from build123d import *
from OCP.BRepFilletAPI import BRepFilletAPI_MakeChamfer
from build123d.topology import SkipClean

# Parameters (mm, degrees)
SALIENTE_EXTRUIR1_DEPTH      = 9
CROQUIS3_R                   = 1.344119186
SALIENTE_EXTRUIR2_DEPTH      = 1
CROQUIS4_R                   = 12.5
CROQUIS4_R_2                 = 1.444119186
SALIENTE_EXTRUIR3_DEPTH      = 3
CROQUIS5_R                   = 1.444119186
SALIENTE_EXTRUIR4_DEPTH      = 2
SALIENTE_EXTRUIR5_START      = -3
CROQUIS6_R                   = 1.625
SALIENTE_EXTRUIR5_DEPTH      = 3
CROQUIS7_R                   = 3.125
CROQUIS7_R_2                 = 1.625
SALIENTE_EXTRUIR6_DEPTH      = 1.75
CROQUIS8_R                   = 3.125
CROQUIS8_R_2                 = 1.625
SALIENTE_EXTRUIR7_DEPTH      = 10
SALIENTE_EXTRUIR8_DEPTH      = 13
SALIENTE_EXTRUIR8_DEPTH_BACK = 7
CROQUIS9_R                   = 2.5
REDONDEO1_R                  = 2.5
CROQUIS11_R                  = 2.5
CROQUIS11_R_2                = 1
SALIENTE_EXTRUIR9_DEPTH      = 10
CHAFL_N1_SIZE                = 2
CHAFL_N1_SIZE2               = 1
CROQUIS10_R                  = 1
CORTAR_EXTRUIR1_DEPTH        = 15


with BuildPart() as part:
    # Croquis2 → Saliente-Extruir1 (new body)
    with BuildSketch(Plane.XY):
        with BuildLine():
            Line((-12.5, 12.5), (12.5, 12.5))
            Line((12.5, 12.5), (12.5, 9.5))
            Line((12.5, 9.5), (9.952027427, 7.563540844))
            ThreePointArc((9.952027427, 7.563540844), (12.5, 0), (9.952027427, -7.563540844))
            Line((9.952027427, -7.563540844), (12.5, -9.5))
            Line((12.5, -9.5), (12.5, -12.5))
            Line((12.5, -12.5), (-12.5, -12.5))
            Line((-12.5, -12.5), (-12.5, -9.5))
            Line((-12.5, -9.5), (-9.952027427, -7.563540844))
            ThreePointArc((-9.952027427, -7.563540844), (-12.5, 0), (-9.952027427, 7.563540844))
            Line((-9.952027427, 7.563540844), (-12.5, 9.5))
            Line((-12.5, 9.5), (-12.5, 12.5))
        make_face()
    extrude(amount=SALIENTE_EXTRUIR1_DEPTH)

    # Croquis3 → Saliente-Extruir2 (add)
    with BuildSketch(Plane(origin=(0, 0, 0), x_dir=(-1, 0, 0), z_dir=(0, 0, -1))):
        Circle(CROQUIS3_R)
    extrude(amount=SALIENTE_EXTRUIR2_DEPTH)



with BuildPart() as body_2:
    # Croquis4 → Saliente-Extruir3 (new body)
    with BuildSketch(Plane(origin=(0, 0, 0), x_dir=(-1, 0, 0), z_dir=(0, 0, -1))):
        Circle(CROQUIS4_R)
        Circle(CROQUIS4_R_2, mode=Mode.SUBTRACT)
    extrude(amount=SALIENTE_EXTRUIR3_DEPTH)

    # Croquis5 → Saliente-Extruir4 (add)
    with BuildSketch(Plane(origin=(0, 0, -3), x_dir=(-1, 0, 0), z_dir=(0, 0, -1))):
        Circle(CROQUIS5_R)
    extrude(amount=-SALIENTE_EXTRUIR4_DEPTH)

    # Croquis6 → Saliente-Extruir5 (add)
    # profile 1 of 2: a face of its own
    with BuildSketch(Plane(origin=(0, 0, -3), x_dir=(-1, 0, 0), z_dir=(0, 0, -1)).offset(SALIENTE_EXTRUIR5_START)):
        with BuildLine():
            Line((-12.478662951, 0.73004859), (-16.792901594, -0.118663584))
            ThreePointArc((-16.792901594, -0.118663584), (-19.255933186, -3.788094791), (-15.586501979, -6.251126382))
            Line((-15.586501979, -6.251126382), (-11.272263337, -5.402414208))
            ThreePointArc((-11.272263337, -5.402414208), (-12.264925596, -2.41279923), (-12.478662951, 0.73004859))
        make_face()
        with Locations((-16.189701787, -3.184894983)):
            Circle(CROQUIS6_R, mode=Mode.SUBTRACT)
    # profile 2 of 2: a face of its own
    with BuildSketch(Plane(origin=(0, 0, -3), x_dir=(-1, 0, 0), z_dir=(0, 0, -1)).offset(SALIENTE_EXTRUIR5_START)):
        with BuildLine():
            Line((15.586501979, 6.251126382), (11.272263337, 5.402414208))
            ThreePointArc((11.272263337, 5.402414208), (12.264925596, 2.41279923), (12.478662951, -0.73004859))
            Line((12.478662951, -0.73004859), (16.792901594, 0.118663584))
            ThreePointArc((16.792901594, 0.118663584), (19.255933186, 3.788094791), (15.586501979, 6.251126382))
        make_face()
        with Locations((16.189701787, 3.184894983)):
            Circle(CROQUIS6_R, mode=Mode.SUBTRACT)
    extrude(amount=SALIENTE_EXTRUIR5_DEPTH)

    # Croquis7 → Saliente-Extruir6 (add)
    # profile 1 of 2: a face of its own
    with BuildSketch(Plane(origin=(0, 0, -3), x_dir=(-1, 0, 0), z_dir=(0, 0, -1))):
        with Locations((-16.189701787, -3.184894983)):
            Circle(CROQUIS7_R)
        with Locations((-16.189701787, -3.184894983)):
            Circle(CROQUIS7_R_2, mode=Mode.SUBTRACT)
    # profile 2 of 2: a face of its own
    with BuildSketch(Plane(origin=(0, 0, -3), x_dir=(-1, 0, 0), z_dir=(0, 0, -1))):
        with Locations((16.189701787, 3.184894983)):
            Circle(CROQUIS7_R)
        with Locations((16.189701787, 3.184894983)):
            Circle(CROQUIS7_R_2, mode=Mode.SUBTRACT)
    extrude(amount=SALIENTE_EXTRUIR6_DEPTH)

    # Croquis8 → Saliente-Extruir7 (add)
    # profile 1 of 2: a face of its own
    with SkipClean():  # the faces are left unmerged after this step: merging them gives an invalid solid
        with BuildSketch(Plane.XY):
            with Locations(Location((-16.189701787, 3.184894983, 0), (0, 0, 180))):
                Circle(CROQUIS8_R)
            with Locations(Location((-16.189701787, 3.184894983, 0), (0, 0, 180))):
                Circle(CROQUIS8_R_2, mode=Mode.SUBTRACT)
        # profile 2 of 2: a face of its own
        with BuildSketch(Plane.XY):
            with Locations(Location((16.189701787, -3.184894983, 0), (0, 0, 180))):
                Circle(CROQUIS8_R)
            with Locations(Location((16.189701787, -3.184894983, 0), (0, 0, 180))):
                Circle(CROQUIS8_R_2, mode=Mode.SUBTRACT)
        extrude(amount=SALIENTE_EXTRUIR7_DEPTH)


with BuildPart() as part_1:
    add(part.part)

    add(body_2.part)  # Saliente-Extruir8 merges body 2
    # Croquis9 → Saliente-Extruir8 (add, two sides: drawn at the far end of the back side and taken through both)
    with BuildSketch(Plane(origin=(0, 12.5, 0), x_dir=(1, 0, 0), z_dir=(0, 1, 0)).offset(-SALIENTE_EXTRUIR8_DEPTH_BACK)):
        with Locations(Location((0, -9, 0), (0, 0, 270))):
            Circle(CROQUIS9_R)
    extrude(amount=SALIENTE_EXTRUIR8_DEPTH + SALIENTE_EXTRUIR8_DEPTH_BACK)

    # Redondeo1
    redondeo1_edges = [part_1.edges().sort_by_distance(p)[0] for p in [
        (1.767766953, 5.5, 10.767766953),
    ]]
    fillet(redondeo1_edges, radius=REDONDEO1_R - 0.0001)  # a hair under: the kernel refuses the full size

    # Croquis11 → Saliente-Extruir9 (add)
    with BuildSketch(Plane.XZ.offset(12.5)):
        with Locations(Location((0, 3, 0), (0, 0, 90))):
            Circle(CROQUIS11_R)
        with Locations(Location((0, 3, 0), (0, 0, 270))):
            Circle(CROQUIS11_R_2, mode=Mode.SUBTRACT)
    extrude(amount=SALIENTE_EXTRUIR9_DEPTH)

    # Chaflán1: one chamfer whose edges measure the first distance from different faces: ONE call of the kernel's chamfer builder (chamfer() names one face for all edges)
    chafl_n1_edges_1 = [part_1.edges().sort_by_distance(p)[0] for p in [
        (0, 25.5, 6.5),
    ]]
    chafl_n1_side_1 = [part_1.faces().sort_by_distance(p)[0] for p in [
        (0, 19, 6.5),
    ]]
    chafl_n1_edges_2 = [part_1.edges().sort_by_distance(p)[0] for p in [
        (0, -22.5, 0.5),
    ]]
    chafl_n1_side_2 = [part_1.faces().sort_by_distance(p)[0] for p in [
        (0, -17.5, 0.5),
    ]]
    chafl_n1 = BRepFilletAPI_MakeChamfer(part_1.part.solid().wrapped)
    for e in chafl_n1_edges_1:
        chafl_n1.Add(CHAFL_N1_SIZE, CHAFL_N1_SIZE2, e.wrapped, chafl_n1_side_1[0].wrapped)  # the first distance lies on this face
    for e in chafl_n1_edges_2:
        chafl_n1.Add(CHAFL_N1_SIZE, CHAFL_N1_SIZE2, e.wrapped, chafl_n1_side_2[0].wrapped)  # the first distance lies on this face
    add(Compound.cast(chafl_n1.Shape()), mode=Mode.REPLACE)

    # Croquis10 → Cortar-Extruir1 (cut)
    with BuildSketch(Plane(origin=(0, 25.5, 0), x_dir=(1, 0, 0), z_dir=(0, 1, 0))):
        with Locations(Location((0, -9, 0), (0, 0, 270))):
            Circle(CROQUIS10_R)
    extrude(amount=-CORTAR_EXTRUIR1_DEPTH, mode=Mode.SUBTRACT)


solid = part_1.part
Design review of the part built by this model. Coordinates are the model's own, in mm. A direction names the side the tool comes from. Give positions to 0.01 mm unless a question says otherwise; leave off trailing zeros. Order: outer loops, then holes, each group sorted by start corner. A loop starts at its lowest first (then second) coordinate and runs counter-clockwise, first axis right, second up.
1. For pin 1 Ø1.5 at (x, y) = (-5, 9) entering from -Z; pin 2 Ø2 at (x, z) = (-8, 1) entering from +Y; pin 3 Ø12 at (x, y) = (-7, 18.5) entering from +Z; pin 4 Ø3 at (x, y) = (-16.19, 3.18) entering from -Z, all flat-tipped, find the tip position at first contact; note any pin that passes through.
Solution:
pin 1: stops at z = -3
pin 2: stops at y = 12.5
pin 3: stops at z = 11.29
pin 4: passes through
2. Add section D-D, the plane y = -10.5. State the section outline as (x, z) points.
Solution:
outline: (-12.5, 0) - (-6.78, 0) - (-6.78, -3) - (6.78, -3) - (6.78, 0) - (12.5, 0) - (12.5, 9) - (-12.5, 9) - close
3. Add section C-C, the plane x = -9. State the section outline as (y, z) points.
Solution:
outline: (-12.5, 0) - (-8.67, 0) - (-8.67, -3) - (8.67, -3) - (8.67, 0) - (12.5, 0) - (12.5, 9) - (-12.5, 9) - close
4. Tool access review of faces 5 (the flat face through (12.8, -2.7, 0)), 6 (the flat face through (11.244, 8.545, 4.437)), 7 (the flat face through (13.46, -5.833, -1.479)), 8 (the flat face through (-13.46, 5.833, -1.479)), 9 (the flat face through (-11.21, 8.52, 4.44)): name each direction out of +Z, -Z, +X, -X, +Y, -Y from which nothing blocks a thin tool from reaching the whole face with its end or side.
Solution:
face 5: +Z
face 6: +Z, -Z, +X
face 7: +Z, -Z, -Y
face 8: +Z, -Z, +Y
face 9: +Z, -Z, -X
5. Add section B-B, the plane y = -19. State the section outline as (x, z) points, then the cut area to 3 significant figures.
Solution:
outline: circle Ø5 at (0, 3); hole circle Ø2 at (0, 3)
area: 16.5 mm2
6. To check wall thickness, follow L1, parallel to Y at x = -10.5, z = 3.5; L2, parallel to X at y = 3, z = 2.25; L3, parallel to X at y = 2, z = 5.75. State the ranges of each line that lie inside material, in increasing order.
Solution:
L1: y = -12.5 to -7.98, -6.78 to 6.78, 7.98 to 12.5
L2: x = -19.31 to -17.8, -14.58 to -13.07, -12.13 to 12.13
L3: x = -19.08 to -17.3, -15.08 to -13.3, -12.34 to 12.34
7. Add section A-A, the plane z = 3. State the section outline as (x, y) points (3 decimals), then the cut area to 3 significant figures.
Solution:
outline: circle Ø6.25 at (-16.19, 3.185); (-12.5, -12.5) - (-2.5, -12.5) - (-2.5, -20.5) - (-1.5, -22.5) - (-1, -22.5) - (-1, -12.5) - (1, -12.5) - (1, -22.5) - (1.5, -22.5) - (2.5, -20.5) - (2.5, -12.5) - (12.5, -12.5) - (12.5, -9.5) - (9.952, -7.564) arc R12.5 ccw to (9.952, 7.564) - (12.5, 9.5) - (12.5, 12.5) - (-12.5, 12.5) - (-12.5, 9.5) - (-9.952, 7.564) arc R12.5 ccw to (-9.952, -7.564) - (-12.5, -9.5) - close; circle Ø6.25 at (16.19, -3.185); hole circle Ø3.25 at (-16.19, 3.185); hole circle Ø3.25 at (16.19, -3.185)
area: 663 mm2
8. Mouldability with a two-part tool opening along Z and no side actions: class faces 1 (the flat face through (-14.61, -0.31, -1.48)), 2 (the flat face through (-13, 2, 0)), 3 (the flat face through (9, 11, 0)), 4 (the cylindrical face through (-0.6, 18.1, 8.2)) as +Z half, -Z half, draft (parallel to the pull), parting line (faces both ways), or undercut.
Solution:
face 1: draft
face 2: +Z half
face 3: -Z half
face 4: undercut
